from build123d import *

# Parameters (mm, degrees)
ESQUISSE1_R        = 1.95
BOSS_EXTRU_1_DEPTH = 5


with BuildPart() as part:
    # Esquisse1 → Boss.-Extru.1 (new body)
    with BuildSketch(Plane.XY):
        Polygon((-10, 25), (-25, 25), (-25, 10), (-30, 10), (-37, 10), (-37, 5), (-35, 5), (-35, 6.5), (-30, 6.5), (-30, 5), (-25, 5), (-25, 0), (-25, -5), (-30, -5), (-30, -6.5), (-35, -6.5), (-35, -5), (-37, -5), (-37, -10), (-30, -10), (-25, -10), (-25, -25), (-10, -25), (-10, -30), (-10, -37), (-5, -37), (-5, -35), (-6.5, -35), (-6.5, -30), (-5, -30), (-5, -25), (0, -25), (5, -25), (5, -30), (6.5, -30), (6.5, -35), (5, -35), (5, -37), (10, -37), (10, -30), (10, -25), (25, -25), (25, -10), (30, -10), (37, -10), (37, -5), (35, -5), (35, -6.5), (30, -6.5), (30, -5), (25, -5), (25, 0), (25, 5), (30, 5), (30, 6.5), (35, 6.5), (35, 5), (37, 5), (37, 10), (30, 10), (25, 10), (25, 25), (10, 25), (10, 30), (10, 37), (5, 37), (5, 35), (6.5, 35), (6.5, 30), (5, 30), (5, 25), (0, 25), (-5, 25), (-5, 30), (-6.5, 30), (-6.5, 35), (-5, 35), (-5, 37), (-10, 37), (-10, 30), align=None)
        with Locations((-22, 0)):
            Circle(ESQUISSE1_R, mode=Mode.SUBTRACT)
        Circle(ESQUISSE1_R, mode=Mode.SUBTRACT)
        with BuildLine():
            Line((15, -21), (-15, -21))
            ThreePointArc((-15, -21), (-21, -15), (-15, -9))
            Line((-15, -9), (15, -9))
            ThreePointArc((15, -9), (21, -15), (15, -21))
        make_face(mode=Mode.SUBTRACT)
        with Locations((22, 0)):
            Circle(ESQUISSE1_R, mode=Mode.SUBTRACT)
        with BuildLine():
            ThreePointArc((-15, 9), (-21, 15), (-15, 21))
            Line((-15, 21), (15, 21))
            ThreePointArc((15, 21), (21, 15), (15, 9))
            Line((15, 9), (-15, 9))
        make_face(mode=Mode.SUBTRACT)
    extrude(amount=BOSS_EXTRU_1_DEPTH)


solid = part.part
Can you work these out from the model? Positions are in its coordinate system, mm. A direction names the side the tool comes from. Round coordinates to 2 decimals unless told otherwise and drop trailing zeros. Write each loop counter-clockwise with the first axis right and the second up, starting at its lowest first coordinate (ties: lowest second). Pieces come first, ordered by that corner, then holes. Notation, with made-up numbers: M -10.75,-12 L 21.25,-12 A26 cw 21.25,5 Z; hole C 83,74.25 d9. An arc over 180 degrees is marked long. Use CSV: the item, a comma, the result in double quotes.
(1) On a 3-axis mill with a long thin cutter (end or side, diameter ignored), from which of +Z, -Z, +X, -X, +Y, -Y can I reach the whole of each face in a straight line? I mean faces 5 (the flat face through (25, 0, 2)), 6 (the flat face through (5, -36, 2)), 7 (the flat face through (25, -18, 2)), 8 (the flat face through (6.5, 33, 2)). Say none if no direction works.
Check values:
face 5,"+Z, -Z, +X"
face 6,"+Z, -Z, -Y"
face 7,"+Z, -Z, +X, -Y"
face 8,"+Z, -Z"
(2) We'd pull the mould along X, two halves only. Please class faces 1 (the flat face through (-10, -31, 2)), 2 (the flat face through (31, -10, 2)), 3 (the flat face through (-5, 27, 2)), 4 (the flat face through (10, 31, 2)): +X half, -X half, draft (parallel to the pull), parting line (faces both ways), or undercut.
Check values:
face 1,"-X half"
face 2,"draft"
face 3,"undercut"
face 4,"+X half"
(3) Imagine slicing it at B-B (x = -22). Write out the boundary of the cut face in (y, z).
Check values:
outline,"M -25,0 L -1.95,0 L -1.95,5 L -25,5 Z; M 1.95,0 L 25,0 L 25,5 L 1.95,5 Z"
(4) Imagine slicing it at A-A (y = 32). Write out the boundary of the cut face in (x, z), plus the area to 3 significant figures.
Check values:
outline,"M -10,0 L -6.5,0 L -6.5,5 L -10,5 Z; M 6.5,0 L 10,0 L 10,5 L 6.5,5 Z"
area,"35.0 mm^2"
(5) I'm going to push flat-ended pins straight in: pin 1 (1 mm diameter, centred on y = 26.5, z = 4, fed in from +X); pin 2 (1.5 mm diameter, centred on x = -26.5, z = 1.5, fed in from +Y); pin 3 (1.5 mm diameter, centred on y = -27, z = 2, fed in from -X). Where does each tip first touch, or does it pass through?
Check values:
pin 1,"x = 10"
pin 2,"y = 10"
pin 3,"x = -10"
(6) I need wall thicknesses on line 1 along Y through (x, z) = (9, 2.25); line 2 along X through (y, z) = (-6, 3.15); line 3 along Y through (x, z) = (-14, 4.15). Which ranges of each line are inside material? Lowest first, please.
Check values:
line 1,"-37 to -21, -9 to 9, 21 to 37"
line 2,"-37 to -35, -30 to 30, 35 to 37"
line 3,"-25 to -21, -9 to 9, 21 to 25"
(7) Imagine slicing it at C-C (x = 11). Write out the boundary of the cut face in (y, z).
Check values:
outline,"M -25,0 L -21,0 L -21,5 L -25,5 Z; M -9,0 L 9,0 L 9,5 L -9,5 Z; M 21,0 L 25,0 L 25,5 L 21,5 Z"
(8) Imagine slicing it at D-D (z = 1.8). Count the separate pieces of the cut face and the enclosed holes in it, plus the area to 3 significant figures.
Check values:
separate pieces,"1"
enclosed holes,"5"
area,"1,940 mm^2"
